```python
from build123d import *
from OCP.BRepFilletAPI import BRepFilletAPI_MakeChamfer

# Parameters (mm, degrees)
SKETCH_1_R          = 55
EXTRUDE_1_DEPTH     = 5
SKETCH_2_R          = 49.9
EXTRUDE_2_DEPTH     = 3
SKETCH_3_W          = 35
SKETCH_3_H          = 30
EXTRUDE_3_DEPTH     = 25
SKETCH_5_R          = 4.1
CUT_EXTRUDE_2_DEPTH = 82.700673192
SKETCH_6_R          = 2.75
CUT_EXTRUDE_3_DEPTH = 85.492603227
BOSS_EXTRUDE1_DEPTH = 5
FILLET1_R           = 10
SKETCH2_W           = 20.25
SKETCH2_H           = 10.35
CUT_EXTRUDE1_DEPTH  = 95.372930441
SKETCH3_W           = 27.9
SKETCH3_H           = 17.5
CUT_EXTRUDE2_DEPTH  = 5
CHAMFER1_SIZE       = 2
CHAMFER1_SIZE2      = 0.535898385
SKETCH4_W           = 35
SKETCH4_H           = 30
CUT_EXTRUDE3_DEPTH  = 12.5
BOSS_EXTRUDE2_START = -2
SKETCH5_W           = 20
SKETCH5_H           = 70
BOSS_EXTRUDE2_DEPTH = 5.325
SKETCH6_R           = 4.1
CUT_EXTRUDE4_DEPTH  = 79.914863161
CUT_EXTRUDE5_DEPTH  = 6.5


with BuildPart() as part:
    # Эскиз1 → Бобышка-Вытянуть1 (new body)
    with BuildSketch(Plane(origin=(0, 0, 0), x_dir=(1, 0, 0), z_dir=(0, 1, 0))):
        with Locations(Location((0, 0, 0), (0, 0, 270))):
            Circle(SKETCH_1_R)
    extrude(amount=EXTRUDE_1_DEPTH)

    # Эскиз2 → Бобышка-Вытянуть2 (add)
    with BuildSketch(Plane(origin=(0, 5, 0), x_dir=(1, 0, 0), z_dir=(0, 1, 0))):
        with Locations(Location((0, 0, 0), (0, 0, 270))):
            Circle(SKETCH_2_R)
    extrude(amount=EXTRUDE_2_DEPTH)

    # Эскиз3 → Бобышка-Вытянуть3 (add)
    with BuildSketch(Plane.XZ):
        Rectangle(SKETCH_3_W, SKETCH_3_H)
    extrude(amount=EXTRUDE_3_DEPTH)

    # Эскиз5 → Вырез-Вытянуть2 (cut, through all)
    with BuildSketch(Plane.XZ):
        with Locations(Location((33.592198598, -32.871936263, 0), (0, 0, 270))):
            Circle(SKETCH_5_R)
        with Locations(Location((-33.591727056, -32.872418125, 0), (0, 0, 270))):
            Circle(SKETCH_5_R)
        with Locations(Location((-33.591727056, 32.872418125, 0), (0, 0, 270))):
            Circle(SKETCH_5_R)
        with Locations(Location((33.483215177, 32.983215177, 0), (0, 0, 270))):
            Circle(SKETCH_5_R)
    extrude(amount=-CUT_EXTRUDE_2_DEPTH, mode=Mode.SUBTRACT)

    # Эскиз6 → Вырез-Вытянуть3 (cut, through all)
    with BuildSketch(Plane(origin=(0, 8, 0), x_dir=(1, 0, 0), z_dir=(0, 1, 0))):
        with Locations(Location((-17.999856554, 19.999999999, 0), (0, 0, 270))):
            Circle(SKETCH_6_R)
    extrude(amount=-CUT_EXTRUDE_3_DEPTH, mode=Mode.SUBTRACT)

    # Sketch1 → Boss-Extrude1 (add)
    with BuildSketch(Plane.XZ):
        with BuildLine():
            Line((55, 0), (55, -31.546703999))
            Line((55, -31.546703999), (45.053362436, -31.546703999))
            ThreePointArc((45.053362436, -31.546703999), (52.454432291, -16.538818973), (55, 0))
        make_face()
    extrude(amount=-BOSS_EXTRUDE1_DEPTH)

    # Fillet1
    # the kernel refuses this fillet: 10 mm, written as the material it takes off along each edge
    with BuildSketch(Plane(origin=(55, -25, -31.546703999), x_dir=(0, 0, 1), z_dir=(0, 1, 0))) as fillet1_piece_1_section:
        with BuildLine():
            CenterArc((FILLET1_R, -FILLET1_R), FILLET1_R, 90, 90)
            Line((0, -FILLET1_R), (0, 0))
            Line((0, 0), (FILLET1_R, 0))
        make_face()
    fillet1_piece_1 = extrude(amount=55, mode=Mode.PRIVATE)
    fillet1_piece_1 = fillet1_piece_1 - Plane(origin=(0, 2.5, 0), x_dir=(0, 0, 1), z_dir=(0, -1, 0)) * Cylinder(55, 150, mode=Mode.PRIVATE)
    add(fillet1_piece_1, mode=Mode.SUBTRACT)

    # Sketch2 → Cut-Extrude1 (cut, through all)
    with BuildSketch(Plane.ZY.offset(17.5)):
        with Locations((0, -12.5)):
            Rectangle(SKETCH2_W, SKETCH2_H)
    extrude(amount=-CUT_EXTRUDE1_DEPTH, mode=Mode.SUBTRACT)

    # Sketch3 → Cut-Extrude2 (cut)
    with BuildSketch(Plane(origin=(0, 8, 0), x_dir=(1, 0, 0), z_dir=(0, 1, 0))):
        with Locations((15.042136476, -5)):
            Rectangle(SKETCH3_W, SKETCH3_H)
    extrude(amount=-CUT_EXTRUDE2_DEPTH, mode=Mode.SUBTRACT)

    # Chamfer1: one chamfer whose edges measure the first distance from different faces: ONE call of the kernel's chamfer builder (chamfer() names one face for all edges)
    chamfer1_edges_1 = [part.edges().sort_by_distance(p)[0] for p in [
        (0.000357897, 8, -49.899999999),
    ]]
    chamfer1_side_1 = [part.faces().sort_by_distance(p)[0] for p in [
        (0.000357897, 6.5, -49.899999999),
    ]]
    chamfer1_edges_2 = [part.edges().sort_by_distance(p)[0] for p in [
        (-49.9, 8, 0),
    ]]
    chamfer1_side_2 = [part.faces().sort_by_distance(p)[0] for p in [
        (-49.9, 6.5, 0),
    ]]
    chamfer1_edges_3 = [part.edges().sort_by_distance(p)[0] for p in [
        (-0.08242255, 8, 49.899931929),
    ]]
    chamfer1_side_3 = [part.faces().sort_by_distance(p)[0] for p in [
        (-0.08242255, 6.5, 49.899931929),
    ]]
    chamfer1_edges_4 = [part.edges().sort_by_distance(p)[0] for p in [
        (49.899931657, 8, 0.082587101),
    ]]
    chamfer1_side_4 = [part.faces().sort_by_distance(p)[0] for p in [
        (49.899931657, 6.5, 0.082587101),
    ]]
    chamfer1 = BRepFilletAPI_MakeChamfer(part.part.solid().wrapped)
    for e in chamfer1_edges_1:
        chamfer1.Add(CHAMFER1_SIZE, CHAMFER1_SIZE2, e.wrapped, chamfer1_side_1[0].wrapped)  # the first distance lies on this face
    for e in chamfer1_edges_2:
        chamfer1.Add(CHAMFER1_SIZE, CHAMFER1_SIZE2, e.wrapped, chamfer1_side_2[0].wrapped)  # the first distance lies on this face
    for e in chamfer1_edges_3:
        chamfer1.Add(CHAMFER1_SIZE, CHAMFER1_SIZE2, e.wrapped, chamfer1_side_3[0].wrapped)  # the first distance lies on this face
    for e in chamfer1_edges_4:
        chamfer1.Add(CHAMFER1_SIZE, CHAMFER1_SIZE2, e.wrapped, chamfer1_side_4[0].wrapped)  # the first distance lies on this face
    add(Compound.cast(chamfer1.Shape()), mode=Mode.REPLACE)

    # Sketch4 → Cut-Extrude3 (cut)
    with BuildSketch(Plane.XZ.offset(25)):
        Rectangle(SKETCH4_W, SKETCH4_H)
    extrude(amount=-CUT_EXTRUDE3_DEPTH, mode=Mode.SUBTRACT)

    # Sketch5 → Boss-Extrude2 (add)
    with BuildSketch(Plane.XZ.offset(7.325).offset(BOSS_EXTRUDE2_START)):
        Rectangle(SKETCH5_W, SKETCH5_H)
    extrude(amount=-BOSS_EXTRUDE2_DEPTH)

    # Sketch6 → Cut-Extrude4 (cut, through all)
    with BuildSketch(Plane.XZ.offset(5.325)):
        with Locations(Location((0, 25, 0), (0, 0, 270))):
            Circle(SKETCH6_R)
        with Locations(Location((0, -25, 0), (0, 0, 270))):
            Circle(SKETCH6_R)
    extrude(amount=-CUT_EXTRUDE4_DEPTH, mode=Mode.SUBTRACT)

    # Sketch7 → Cut-Extrude5 (cut)
    with BuildSketch(Plane(origin=(0, 8, 0), x_dir=(1, 0, 0), z_dir=(0, 1, 0))):
        Polygon((0, -32.5), (6.495190528, -28.75), (6.495190528, -21.25), (0, -17.5), (-6.495190528, -21.25), (-6.495190528, -28.75), align=None)
        Polygon((0, 17.5), (6.495190528, 21.25), (6.495190528, 28.75), (0, 32.5), (-6.495190528, 28.75), (-6.495190528, 21.25), align=None)
    extrude(amount=-CUT_EXTRUDE5_DEPTH, mode=Mode.SUBTRACT)


solid = part.part
```
CAD build for the part. Positions are in the model's coordinates, mm. A direction names the side the tool comes from. Give positions to 0.01 mm unless a question says otherwise; leave off trailing zeros. Loops run counter-clockwise (first coordinate to the right, second up) from the corner with the lowest first, then second, coordinate; pieces in that order, holes last. Notation, with made-up numbers: (10.5, 10) - (16.5, 10) arc R32 cw to (16.5, 43) - close; hole circle Ø2 at (-22, 88.25). An arc over 180 degrees is marked (long way). Put each result on its own line as item: value.
Q1. Slice it at A-A (y = -9.25). Give the cut face in (x, z) (3 decimals), plus the area to 3 significant figures.
Filled in:
outline: (-17.5, -15) - (17.5, -15) - (17.5, -10.125) - (-17.5, -10.125) - close; (-17.5, 10.125) - (17.5, 10.125) - (17.5, 15) - (-17.5, 15) - close
area: 341 mm²
Q2. Probe line 1 along Z through (x, y) = (-6, 4); line 2 along X through (y, z) = (-1.5, -25); line 3 along Z through (x, y) = (-37, 1.75). List the from-to ranges inside material, lowest first.
Filled in:
line 1: z = -54.67 to -29.04, -20.96 to 20.96, 29.04 to 54.67
line 2: x = -10 to -4.1, 4.1 to 10
line 3: z = -40.69 to -35.15, -30.59 to 30.59, 35.15 to 40.69
Q3. Tool access for faces 5 (the face through (10, -3, 25)), 6 (the face through (-17.5, -5, 0)), 7 (the face through (10, -3, -25)), 8 (the face through (3.29, 4.8, 19.4)), 9 (the face through (0.515, 5.493, -49.897)): list every direction of +Z, -Z, +X, -X, +Y, -Y with a clear straight run to the whole face (end or side of a thin tool).
Filled in:
face 5: +Z, +X, -Y
face 6: +Z, -Z, -X, -Y
face 7: -Z, +X, -Y
face 8: +Y
face 9: -Z, +Y
Q4. Mould opens along Z. For faces 1 (the face through (-49.898, 5.493, -0.499)), 2 (the face through (0.51, 7.681, -49.447)), 3 (the face through (29.846, 3.944, 31.091)), 4 (the face through (-10, -3, 25)) say: pulls with the +Z half, pulls with the -Z half, needs draft (parallel to the pull), parting line crosses it, or undercut.
Filled in:
face 1: parting line crosses it
face 2: pulls with the -Z half
face 3: undercut
face 4: needs draft
Q5. Flat gauge pins, fed straight in: pin 1 (1.6 mm diameter, centred on y = -2.5, z = 26, fed in from +X); pin 2 (5 mm diameter, centred on y = 2, z = -39, fed in from -X); pin 3 (1.5 mm diameter, centred on y = 5, z = 2.5, fed in from -X); pin 4 (5 mm diameter, centred on x = -18, z = -20, fed in from -Y). Where does each tip first touch, or does it go through?
Filled in:
pin 1: stops at x = 10
pin 2: stops at x = -41.14
pin 3: stops at x = -54.97
pin 4: passes through
